from build123d import *

# Parameters (mm, degrees)
PAD_DEPTH = 10


with BuildPart() as part:
    # CopySketch029 → Pad (new body)
    with BuildSketch(Plane.XY):
        with BuildLine():
            Line((-2.377208, 3.65), (-5.646878, 6.91967))
            ThreePointArc((-5.116548, 8.2), (-5.809457, 7.737013), (-5.646878, 6.91967))
            Line((-5.116548, 8.2), (-2.5, 8.2))
            Line((-2.5, 9.5), (-2.5, 8.2))
            ThreePointArc((-2.5, 9.5), (-2.646447, 9.853553), (-3, 10))
            Line((-3, 10), (-8, 10))
            ThreePointArc((-8, 10), (-9.414214, 9.414214), (-10, 8))
            Line((-10, 8), (-10, 3))
            ThreePointArc((-10, 3), (-9.853553, 2.646447), (-9.5, 2.5))
            Line((-9.5, 2.5), (-8.2, 2.5))
            Line((-8.2, 2.5), (-8.2, 5.116548))
            ThreePointArc((-6.91967, 5.646878), (-7.737013, 5.809457), (-8.2, 5.116548))
            Line((-6.91967, 5.646878), (-3.65, 2.377208))
            Line((-3.65, 2.377208), (-3.65, 0.177208))
            Line((-3.65, 0.177208), (-3.45, 0))
            Line((-3.45, 0), (-2.15, 0))
            ThreePointArc((0, 2.15), (-1.52028, 1.52028), (-2.15, 0))
            Line((0, 3.45), (0, 2.15))
            Line((-0.177208, 3.65), (0, 3.45))
            Line((-0.177208, 3.65), (-2.377208, 3.65))
        make_face()
        with BuildLine():
            Line((2.377208, 3.65), (5.646878, 6.91967))
            ThreePointArc((5.646878, 6.91967), (5.809457, 7.737013), (5.116548, 8.2))
            Line((5.116548, 8.2), (2.5, 8.2))
            Line((2.5, 9.5), (2.5, 8.2))
            ThreePointArc((3, 10), (2.646447, 9.853553), (2.5, 9.5))
            Line((3, 10), (8, 10))
            ThreePointArc((10, 8), (9.414214, 9.414214), (8, 10))
            Line((10, 8), (10, 3))
            ThreePointArc((9.5, 2.5), (9.853553, 2.646447), (10, 3))
            Line((9.5, 2.5), (8.2, 2.5))
            Line((8.2, 2.5), (8.2, 5.116548))
            ThreePointArc((8.2, 5.116548), (7.737013, 5.809457), (6.91967, 5.646878))
            Line((6.91967, 5.646878), (3.65, 2.377208))
            Line((3.65, 2.377208), (3.65, 0.177208))
            Line((3.65, 0.177208), (3.45, 0))
            Line((3.45, 0), (2.15, 0))
            ThreePointArc((2.15, 0), (1.52028, 1.52028), (0, 2.15))
            Line((0, 3.45), (0, 2.15))
            Line((0.177208, 3.65), (0, 3.45))
            Line((0.177208, 3.65), (2.377208, 3.65))
        make_face()
        with BuildLine():
            Line((-2.377208, -3.65), (-5.646878, -6.91967))
            ThreePointArc((-5.646878, -6.91967), (-5.809457, -7.737013), (-5.116548, -8.2))
            Line((-5.116548, -8.2), (-2.5, -8.2))
            Line((-2.5, -9.5), (-2.5, -8.2))
            ThreePointArc((-3, -10), (-2.646447, -9.853553), (-2.5, -9.5))
            Line((-3, -10), (-8, -10))
            ThreePointArc((-10, -8), (-9.414214, -9.414214), (-8, -10))
            Line((-10, -8), (-10, -3))
            ThreePointArc((-9.5, -2.5), (-9.853553, -2.646447), (-10, -3))
            Line((-9.5, -2.5), (-8.2, -2.5))
            Line((-8.2, -2.5), (-8.2, -5.116548))
            ThreePointArc((-8.2, -5.116548), (-7.737013, -5.809457), (-6.91967, -5.646878))
            Line((-6.91967, -5.646878), (-3.65, -2.377208))
            Line((-3.65, -2.377208), (-3.65, -0.177208))
            Line((-3.65, -0.177208), (-3.45, 0))
            Line((-3.45, 0), (-2.15, 0))
            ThreePointArc((-2.15, 0), (-1.52028, -1.52028), (0, -2.15))
            Line((0, -3.45), (0, -2.15))
            Line((-0.177208, -3.65), (0, -3.45))
            Line((-0.177208, -3.65), (-2.377208, -3.65))
        make_face()
        with BuildLine():
            Line((2.377208, -3.65), (5.646878, -6.91967))
            ThreePointArc((5.116548, -8.2), (5.809457, -7.737013), (5.646878, -6.91967))
            Line((5.116548, -8.2), (2.5, -8.2))
            Line((2.5, -9.5), (2.5, -8.2))
            ThreePointArc((2.5, -9.5), (2.646447, -9.853553), (3, -10))
            Line((3, -10), (8, -10))
            ThreePointArc((8, -10), (9.414214, -9.414214), (10, -8))
            Line((10, -8), (10, -3))
            ThreePointArc((10, -3), (9.853553, -2.646447), (9.5, -2.5))
            Line((9.5, -2.5), (8.2, -2.5))
            Line((8.2, -2.5), (8.2, -5.116548))
            ThreePointArc((6.91967, -5.646878), (7.737013, -5.809457), (8.2, -5.116548))
            Line((6.91967, -5.646878), (3.65, -2.377208))
            Line((3.65, -2.377208), (3.65, -0.177208))
            Line((3.65, -0.177208), (3.45, 0))
            Line((3.45, 0), (2.15, 0))
            ThreePointArc((0, -2.15), (1.52028, -1.52028), (2.15, 0))
            Line((0, -3.45), (0, -2.15))
            Line((0.177208, -3.65), (0, -3.45))
            Line((0.177208, -3.65), (2.377208, -3.65))
        make_face()
    extrude(amount=PAD_DEPTH)


solid = part.part
Input: part model. Units: mm. Frame: model coordinates. A direction names the side the tool comes from. Coordinates: 2 decimals unless noted, no trailing zeros. Order: outer loops, then holes, each group sorted by start corner. A loop starts at its lowest first (then second) coordinate and runs counter-clockwise, first axis right, second up. Notation, with made-up numbers: M -34.75,6.5 L -22.75,6.5 A12 ccw -22.75,12.5 Z; hole C -24,-21.75 d1. An arc over 180 degrees is marked long. One line per question, with ' | ' between items.
Item 1: Draft query along X for faces 5 (the flat face through (9, 2.5, 5)), 6 (the cylindrical face through (-9.43, -9.4, 4.93)), 7 (the cylindrical face through (5.805, -7.748, 4.93)). Return one class per face: released by +X, released by -X, zero draft, split by the parting line, or undercut.
Geometry results:
face 5: zero draft | face 6: released by -X | face 7: undercut
Item 2: Section C-C (y = -4.5). Output: boundary loops of the cut face in (x, z), then the cut area to 3 significant figures.
Geometry results:
outline: M -10,0 L -8.2,0 L -8.2,10 L -10,10 Z; M -5.77,0 L -3.23,0 L -3.23,10 L -5.77,10 Z; M 3.23,0 L 5.77,0 L 5.77,10 L 3.23,10 Z; M 8.2,0 L 10,0 L 10,10 L 8.2,10 Z | area: 86.9 mm^2
Item 3: Reachability of faces 1 (the flat face through (2.5, -9, 5)), 2 (the flat face through (3.65, -1, 5)), 3 (the flat face through (5.308, -4.035, 4.93)), 4 (the flat face through (1, 3.65, 5)) from +Z, -Z, +X, -X, +Y, -Y: full face, straight path, thin tool, end or side. Return the list, or none.
Geometry results:
face 1: +Z, -Z, -Y | face 2: +Z, -Z, +X | face 3: +Z, -Z | face 4: +Z, -Z, +Y
Item 4: Ray query, line 1 along X through (y, z) = (2.75, 7.25); line 2 along X through (y, z) = (3.75, 8); line 3 along X through (y, z) = (5.25, 1). Return the intervals inside material, ascending.
Geometry results:
line 1: x = -9.93 to -8.2, -4.02 to 4.02, 8.2 to 9.93 | line 2: x = -10 to -8.2, -5.02 to -2.48, 2.48 to 5.02, 8.2 to 10 | line 3: x = -10 to -8.19, -6.52 to -3.98, 3.98 to 6.52, 8.19 to 10
Item 5: Pin query (flat end, axial travel): pin 1 (1 mm diameter, centred on y = -9, z = 6.5, fed in from -X); pin 2 (0.7 mm diameter, centred on x = 1.5, z = 3, fed in from +Y); pin 3 (1.5 mm diameter, centred on x = -1, z = 2.5, fed in from -Y). Return the tip coordinate at first contact, or that it passes through.
Geometry results:
pin 1: stops at x = -9.94 | pin 2: stops at y = 3.65 | pin 3: stops at y = -3.65
Item 6: Section A-A (x = -8.5). Output: boundary loops of the cut face in (y, z).
Geometry results:
outline: M -9.94,0 L -2.5,0 L -2.5,10 L -9.94,10 Z; M 2.5,0 L 9.94,0 L 9.94,10 L 2.5,10 Z
